Source: CAD feature listing. Evaluate the final solid. Frame: model axes, mm. Face numbers are marked on the shaded views. Give positions to 0.01 mm unless a question says otherwise; leave off trailing zeros. Write each loop counter-clockwise with the first axis right and the second up, starting at its lowest first coordinate (ties: lowest second). Pieces come first, ordered by that corner, then holes. Notation, with made-up numbers: (89, 0) -> (107, 0) arc R24 ccw to (107, 26) -> close; hole circle Ø9 at (1, 10.25). An arc over 180 degrees is marked (long way). Answer as a JSON object with one key per item and string values. Group by question number.
Item 1: Section query B-B on z = 4.75. Return the cut outline in (x, y) (1 decimal).
Item 2: First-contact query: pin 1 Ø1.5 at (x, z) = (-9, 3) entering from -Y; pin 2 Ø3 at (y, z) = (-6, 7) entering from +X; pin 3 Ø1 at (x, z) = (7.5, 7) entering from +Y. Flat tips, straight axial feed; report the tip coordinate or a pass-through.
Item 3: Ray query, probe 1 along Y at (x, z) = (0, 4.5); probe 2 along X at (y, z) = (-3.5, 9.25); probe 3 along Y at (x, z) = (4.5, 4.75). Return the intervals inside material, ascending. Write a range as from..to.
Item 4: Section query A-A on x = 0. Return the cut outline in (y, z).
Item 5: Pull-direction query (Y, two-part tool) for the marked faces 1, 2 and 3; classes: pulls with the +Y half, pulls with the -Y half, needs draft (parallel to the pull), parting line crosses it, or undercut.
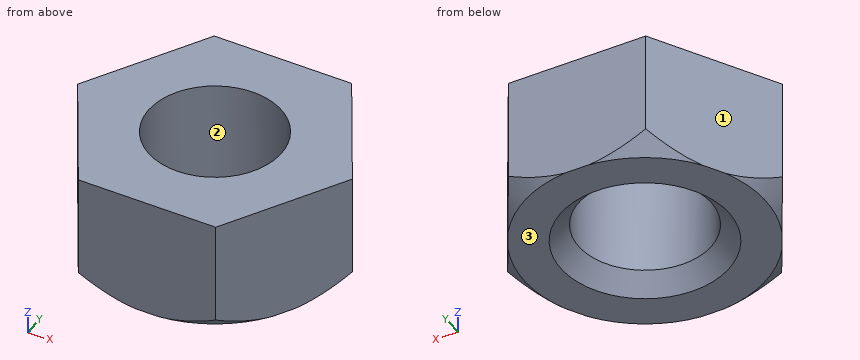
Autodesk Fusion 360 part; units mm, degrees
sketch "Sketch1" plane through (0, 0, 0) normal (0, 0, 1) x (1, 0, 0) in component "nut"
  line L0 (11.547, 0) -> (5.7735, 10)
  line L1 (5.7735, 10) -> (-5.7735, 10)
  line L2 (-5.7735, 10) -> (-11.547, 0)
  line L3 (-11.547, 0) -> (-5.7735, -10)
  line L4 (-5.7735, -10) -> (5.7735, -10)
  line L5 (5.7735, -10) -> (11.547, 0)
  dimension "d1" = 10
extrude "Extrude1" add sketch "Sketch1" along normal blind 10 in component "nut"
sketch "Sketch2" plane through (0, 0, 0) normal (0, 1, 0) x (1, 0, 0) in component "nut"
  line L0 (11.547, -10) -> (10.047, -10)
  line L1 (10.047, -10) -> (11.547, -8.5)
  line L2 (11.547, -8.5) -> (11.547, -10)
  point P0 (11.547, -10)
  dimension "d4" = 1.5
revolve "Revolve1" cut sketch "Sketch2" angle 360 about axis through (0, 0, 1.75) along (0, 0, 1) in component "nut"
hole "Hole1" at (0, 0, 10) direction (0, 0, -1) diameter 11.035 end through all countersink diameter 14 countersink angle 90 in component "nut"
ref_plane "WorkPlane1" through (0, 0, 5) normal (0, 0, 1) x (1, 0, 0) in component "nut"
mirror "Mirror1" about plane through (0, 0, 5) normal (0, 0, 1) of "Extrude1", "Revolve1", "Hole1" in component "nut"
component "nut" placed x (1, 0, 0) y (0, 1, 0) z (0, 0, 1) at (0, 0, 0)
Worked answers:
{
 "1": {"outline": "(-11.5, 0) -> (-5.8, -10) -> (5.8, -10) -> (11.5, 0) -> (5.8, 10) -> (-5.8, 10) -> close; hole circle Ø11 at (0, 0)"},
 "2": {"pin 1": "y = -5.71", "pin 2": "x = 8.95", "pin 3": "y = 7.88"},
 "3": {"probe 1": "-10..-5.52, 5.52..10", "probe 2": "-9.53..-4.27, 4.27..9.53", "probe 3": "-10..-3.19, 3.19..10"},
 "4": {"outline": "(-10, 0) -> (-7, 0) -> (-5.52, 1.48) -> (-5.52, 10) -> (-10, 10) -> close; (5.52, 1.48) -> (7, 0) -> (10, 0) -> (10, 10) -> (5.52, 10) -> close"},
 "5": {"face 1": "pulls with the +Y half", "face 2": "undercut", "face 3": "needs draft"}
}
